from build123d import *

# Parameters (mm, degrees)
F0_W     = 83.4575
F0_H     = 24.77125
F0_H_2   = 83.4575
F0_R     = 1
F0_R_2   = 33
F0_R_3   = 1.5
F1_DEPTH = 1
F2_DEPTH = 2
F3_ANGLE = 90


with BuildPart() as f1:
    # F0 (on Top) → F1 (new body)
    with BuildSketch(Plane.XY):
        with Locations((0, 54.114375)):
            Rectangle(F0_W, F0_H)
        with Locations((0, -54.114375)):
            Rectangle(F0_W, F0_H)
        Rectangle(F0_W, F0_H_2)
        with Locations((-35.241835, -5.300909)):
            Circle(F0_R, mode=Mode.SUBTRACT)
        with Locations((-21.911398, -28.106533)):
            Circle(F0_R, mode=Mode.SUBTRACT)
        with Locations((-28.14937, -21.856339)):
            Circle(F0_R, mode=Mode.SUBTRACT)
        with Locations((-32.853084, -13.811641)):
            Circle(F0_R, mode=Mode.SUBTRACT)
        with Locations((12.550777, -33.355128)):
            Circle(F0_R, mode=Mode.SUBTRACT)
        with Locations((21.307442, -28.567105)):
            Circle(F0_R, mode=Mode.SUBTRACT)
        with Locations((28.306502, -21.652449)):
            Circle(F0_R, mode=Mode.SUBTRACT)
        with Locations((33.0647, -13.297075)):
            Circle(F0_R, mode=Mode.SUBTRACT)
        with Locations((35.280626, -5.036269)):
            Circle(F0_R, mode=Mode.SUBTRACT)
        with Locations((-35.433602, 3.81398)):
            Circle(F0_R, mode=Mode.SUBTRACT)
        with Locations((-33.27858, 12.752359)):
            Circle(F0_R, mode=Mode.SUBTRACT)
        with Locations((-28.561056, 21.31555)):
            Circle(F0_R, mode=Mode.SUBTRACT)
        with Locations((-21.972067, 28.059131)):
            Circle(F0_R, mode=Mode.SUBTRACT)
        with Locations((-13.864813, 32.83068)):
            Circle(F0_R, mode=Mode.SUBTRACT)
        Circle(F0_R_2, mode=Mode.SUBTRACT)
        with Locations((32.911723, 13.671321)):
            Circle(F0_R, mode=Mode.SUBTRACT)
        with Locations((28.498819, 21.398689)):
            Circle(F0_R, mode=Mode.SUBTRACT)
        with Locations((21.63808, 28.317487)):
            Circle(F0_R, mode=Mode.SUBTRACT)
        with Locations((35.335113, 4.638577)):
            Circle(F0_R, mode=Mode.SUBTRACT)
        with Locations((6.526564, 35.035561)):
            Circle(F0_R_3, mode=Mode.SUBTRACT)
    extrude(amount=F1_DEPTH)

    # F0 (on Top) → F2 (join)
    with BuildSketch(Plane.XY):
        Circle(F0_R_2)
        with Locations((-13.864813, 32.83068)):
            Circle(F0_R)
        with Locations((-21.972067, 28.059131)):
            Circle(F0_R)
        with Locations((-28.561056, 21.31555)):
            Circle(F0_R)
        with Locations((-33.27858, 12.752359)):
            Circle(F0_R)
        with Locations((-35.433602, 3.81398)):
            Circle(F0_R)
        with Locations((-35.241835, -5.300909)):
            Circle(F0_R)
        with Locations((-32.853084, -13.811641)):
            Circle(F0_R)
        with Locations((-28.14937, -21.856339)):
            Circle(F0_R)
        with Locations((-21.911398, -28.106533)):
            Circle(F0_R)
        with Locations((12.550777, -33.355128)):
            Circle(F0_R)
        with Locations((21.307442, -28.567105)):
            Circle(F0_R)
        with Locations((28.306502, -21.652449)):
            Circle(F0_R)
        with Locations((33.0647, -13.297075)):
            Circle(F0_R)
        with Locations((35.280626, -5.036269)):
            Circle(F0_R)
        with Locations((35.335113, 4.638577)):
            Circle(F0_R)
        with Locations((32.911723, 13.671321)):
            Circle(F0_R)
        with Locations((28.498819, 21.398689)):
            Circle(F0_R)
        with Locations((21.63808, 28.317487)):
            Circle(F0_R)
        with Locations((6.526564, 35.035561)):
            Circle(F0_R_3)
    extrude(amount=F2_DEPTH)


with BuildPart() as f1_1:
    # F3: moved
    add(f1.part.rotate(Axis((0, 0, 2), (0, 0, 1)), F3_ANGLE))


solid = f1_1.part
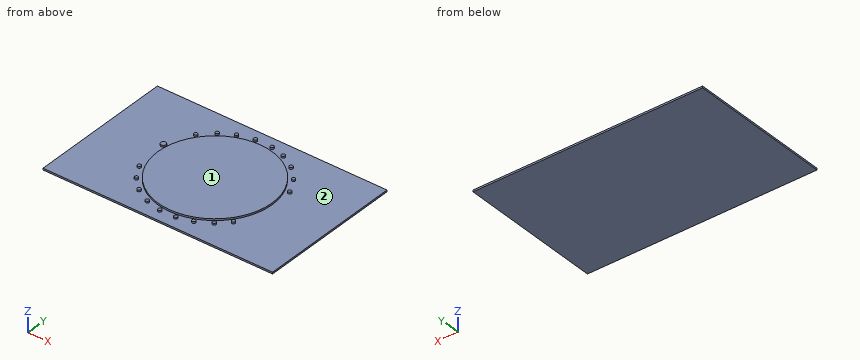
Read the model definition and answer for the solid it produces. Units are mm, in the model's axes. Face numbers are marked on the shaded views. A direction names the side the tool comes from. Give positions to 0.01 mm unless a question says otherwise; leave off trailing zeros. Loops run counter-clockwise (first coordinate to the right, second up) from the corner with the lowest first, then second, coordinate; pieces in that order, holes last. Notation, with made-up numbers: (-39, 37.25) - (-16, 37.25) arc R26 cw to (-16, 70.25) - close; hole circle Ø11 at (18, 43). An arc over 180 degrees is marked (long way). Answer as CSV lines item,"result". Start each with the question number.
1) Find section D-D (x = -54.5). Write down the section's boundary in (y, z), then the cut area to 3 significant figures.
2) Find section A-A (z = 1.4). State how many separate pieces and enclosed holes the cut face has, then the cut area to 3 significant figures.
3) Find section C-C (x = 0). Write down the section's boundary in (y, z), then the cut area to 3 significant figures.
4) Which of the six approach directions +Z, -Z, +X, -X, +Y, -Y give full straight-line access (tool end or side, diameter ignored) to the marked faces 1 and 2?
5) Straight lines are drawn through the part: L1, parallel to X at y = 29, z = 1.1; L2, parallel to Z at x = 52, y = -19; L3, parallel to X at y = -26, z = 1.35. For each, find the intervals that lie inside material, in ascending order. Write a range as from..to.
6) Find section B-B (y = 0). Write down the section's boundary in (x, z), then the cut area to 3 significant figures.
Findings below:
1,outline,"(-41.73, 0) - (41.73, 0) - (41.73, 1) - (-41.73, 1) - close"
1,area,"83.5 mm^2"
2,separate pieces,"20"
2,enclosed holes,"0"
2,area,"3,480 mm^2"
3,outline,"(-41.73, 0) - (41.73, 0) - (41.73, 1) - (33, 1) - (33, 2) - (-33, 2) - (-33, 1) - (-41.73, 1) - close"
3,area,"149 mm^2"
4,face 1,"+Z, +X, -X, +Y, -Y"
4,face 2,"+Z"
5,L1,"-22.26..-20.53, -15.75..15.75, 20.93..22.37"
5,L2,"0..1"
5,L3,"-20.32..20.32"
6,outline,"(-66.5, 0) - (66.5, 0) - (66.5, 1) - (33, 1) - (33, 2) - (-33, 2) - (-33, 1) - (-66.5, 1) - close"
6,area,"199 mm^2"
